Read the model definition and answer for the solid it produces. Units are mm, in the model's axes. A direction names the side the tool comes from. Give positions to 0.01 mm unless a question says otherwise; leave off trailing zeros. Write each loop counter-clockwise with the first axis right and the second up, starting at its lowest first coordinate (ties: lowest second). Pieces come first, ordered by that corner, then holes. Notation, with made-up numbers: (77, -8) - (130, -8) arc R27 cw to (130, 29) - close; hole circle Ø7 at (31, 62). An arc over 180 degrees is marked (long way). Use CSV: the item, a comma, the result in double quotes. Start each with the question number.
from build123d import *

# Parameters (mm, degrees)
SKETCH1_W           = 400
SKETCH1_H           = 300
BOSS_EXTRUDE1_DEPTH = 1010


with BuildPart() as part:
    # Sketch1 → Boss-Extrude1 (new body)
    with BuildSketch(Plane.XZ.offset(4290)):
        with Locations((-200, 150)):
            Rectangle(SKETCH1_W, SKETCH1_H)
    extrude(amount=BOSS_EXTRUDE1_DEPTH)

    # Sketch2 → Loft1 section 0
    with BuildSketch(Plane(origin=(0, 0, -207.664317166), x_dir=(-1, 0, 0), z_dir=(0, 0, -1))):
        with BuildLine():
            Line((400, -5300), (0, -5300))
            Line((0, -5300), (0, -4420))
            Line((0, -4420), (400, -4420))
            Line((400, -4420), (400, -5300))
        make_face()
    # Sketch4 → Loft1 section 1
    with BuildSketch(Plane(origin=(0, 0, 0), x_dir=(-1, 0, 0), z_dir=(0, 0, -1))):
        with BuildLine():
            Line((0, -5300), (400, -5300))
            Line((400, -5300), (400, -4420))
            Line((400, -4420), (0, -4420))
            Line((0, -4420), (0, -5300))
        make_face()
    loft()


solid = part.part
(1) The part is cut by section C-C on z = -63.5. Write down the section's boundary in (x, y).
(2) The part is cut by section B-B on y = -4410. Write down the section's boundary in (x, z).
(3) The part is cut by section A-A on x = -79. Write down the section's boundary in (y, z), plus the area to 3 significant figures.
(4) Which of the six approach directions +Z, -Z, +X, -X, +Y, -Y give full straight-line access (tool end or side, diameter ignored) to faces 1 (the face through (-197, -4420, -102)), 2 (the face through (0, -4802, 50))?
(5) Consider probe 1 along Y at (x, z) = (-230, -79.5). Determine where the line is inside the solid, lowest interval first.
Reported:
1,outline,"(-400, -5300) - (0, -5300) - (0, -4420) - (-400, -4420) - close"
2,outline,"(-400, 0) - (0, 0) - (0, 300) - (-400, 300) - close"
3,outline,"(-5300, -207.66) - (-4420, -207.66) - (-4420, 0) - (-4290, 0) - (-4290, 300) - (-5300, 300) - close"
3,area,"486,000 mm²"
4,face 1,"-Z, +X, -X, +Y"
4,face 2,"+Z, -Z, +X, +Y, -Y"
5,probe 1,"-5300 to -4420"
